Source: CAD feature listing. Evaluate the final solid. Frame: model axes, mm. Coordinates: 2 decimals unless noted, no trailing zeros. Loops run counter-clockwise (first coordinate to the right, second up) from the corner with the lowest first, then second, coordinate; pieces in that order, holes last. Notation, with made-up numbers: (-30, 82.5) -> (-9, 82.5) arc R22 cw to (-9, 102.5) -> close; hole circle Ø8 at (-18, 63). An arc over 180 degrees is marked (long way). One line per question, with ' | ' between items. Start each with the question number.
```python
from build123d import *

# Parameters (mm, degrees)
SKETCH1_W           = 25
SKETCH1_H           = 25
BOSS_EXTRUDE1_DEPTH = 2
SKETCH4_R           = 1.125
BOSS_EXTRUDE3_DEPTH = 0.7
SKETCH5_W           = 21.3
SKETCH5_H           = 21.3
BOSS_EXTRUDE4_DEPTH = 0.01
FILLET1_R           = 0.7
CHAMFER1_SIZE       = 0.5
CUT_EXTRUDE1_DEPTH  = 18.790446875
SKETCH7_R           = 0.4
BOSS_EXTRUDE5_DEPTH = 2


with BuildPart() as part:
    # Sketch1 → Boss-Extrude1 (new body)
    with BuildSketch(Plane.XY):
        Rectangle(SKETCH1_W, SKETCH1_H)
    extrude(amount=BOSS_EXTRUDE1_DEPTH)

    # Sketch4 → Boss-Extrude3 (add)
    with BuildSketch(Plane.XY.offset(2)):
        with Locations((0, 2.5)):
            Circle(SKETCH4_R)
    extrude(amount=BOSS_EXTRUDE3_DEPTH)

    # Sketch5 → Boss-Extrude4 (add)
    with BuildSketch(Plane.XY.offset(2)):
        Rectangle(SKETCH5_W, SKETCH5_H)
    extrude(amount=BOSS_EXTRUDE4_DEPTH)

    # Fillet1
    # the kernel refuses this fillet: 0.7 mm, written as the material it adds along each edge
    with BuildSketch(Plane(origin=(0, 2.5, 2.01), x_dir=(1, 0, 0), z_dir=(0, 1, 0))) as fillet1_piece_1_section:
        with BuildLine():
            CenterArc((1.125 + FILLET1_R, -FILLET1_R), FILLET1_R, 90, 90)
            Line((1.125, -FILLET1_R), (1.125, 0))
            Line((1.125, 0), (1.125 + FILLET1_R, 0))
        make_face()
    fillet1_piece_1 = revolve(axis=Axis((0, 2.5, 2.01), (0, 0, -1)), mode=Mode.PRIVATE)
    fillet1_piece_1 = split(fillet1_piece_1, bisect_by=Plane(origin=(-1.326537578, 2.5, 2.7), z_dir=(0, 0, -1)), keep=Keep.TOP, mode=Mode.PRIVATE)
    add(fillet1_piece_1)

    # Chamfer1
    chamfer1_edges = [part.edges().sort_by_distance(p)[0] for p in [
        (-10.65, -10.65, 2.005),
        (10.65, 10.65, 2.005),
    ]]
    chamfer(chamfer1_edges, length=CHAMFER1_SIZE)

    # Sketch6 → Cut-Extrude1 (cut, through all)
    with BuildSketch(Plane.XY.offset(2)):
        with BuildLine():
            Line((12.5, 9.98277308), (12.5, 12.5))
            Line((12.5, 12.5), (9.98277308, 12.5))
            ThreePointArc((9.98277308, 12.5), (11.762721305, 11.762721305), (12.5, 9.98277308))
        make_face()
        with BuildLine():
            Line((-9.98277308, 12.5), (-12.5, 12.5))
            Line((-12.5, 12.5), (-12.5, 9.98277308))
            ThreePointArc((-12.5, 9.98277308), (-11.762721305, 11.762721305), (-9.98277308, 12.5))
        make_face()
        with BuildLine():
            Line((-12.5, -9.98277308), (-12.5, -12.5))
            Line((-12.5, -12.5), (-9.98277308, -12.5))
            ThreePointArc((-9.98277308, -12.5), (-11.762721305, -11.762721305), (-12.5, -9.98277308))
        make_face()
        with BuildLine():
            Line((12.5, -9.98277308), (12.5, -12.5))
            Line((12.5, -12.5), (9.98277308, -12.5))
            ThreePointArc((9.98277308, -12.5), (11.762721305, -11.762721305), (12.5, -9.98277308))
        make_face()
    extrude(amount=-CUT_EXTRUDE1_DEPTH, mode=Mode.SUBTRACT)

    # Sketch7 → Boss-Extrude5 (add)
    with BuildSketch(Plane(origin=(0, 0, 0), x_dir=(-1, 0, 0), z_dir=(0, 0, -1))):
        with Locations(Location((0, 2.5, 0), (0, 0, 180))):
            Circle(SKETCH7_R)
    extrude(amount=BOSS_EXTRUDE5_DEPTH)


solid = part.part
```
(1) Cut plane A-A, the plane y = 2.5. Return the cut outline in (x, z) (3 decimals).
(2) Cut plane C-C, the plane z = -1.15. Return the cut outline in (x, y), and give its area (3 significant figures).
(3) Cut plane B-B, the plane x = 0. Return the cut outline in (y, z) (3 decimals), and give its area (3 significant figures).
(4) Contact query for a flat-ended pin moving along its axis: pin 1 Ø6 at (x, y) = (2.5, -8) entering from -Z. Output: stop coordinate, or through.
(5) Ray query, L1, parallel to Z at x = -3.75, y = 2.5; L2, parallel to Z at x = 0.5, y = 1.75; L3, parallel to X at y = 10.5, z = 0.3. Return the intervals inside material, ascending.
Here are the results:
1) outline: (-12.5, 0) -> (-0.4, 0) -> (-0.4, -2) -> (0.4, -2) -> (0.4, 0) -> (12.5, 0) -> (12.5, 2) -> (10.65, 2) -> (10.65, 2.01) -> (1.825, 2.01) arc R0.7 cw to (1.125, 2.7) -> (-1.125, 2.7) arc R0.7 cw to (-1.825, 2.01) -> (-10.65, 2.01) -> (-10.65, 2) -> (-12.5, 2) -> close
2) outline: circle Ø0.8 at (0, 2.5) | area: 0.503 mm2
3) outline: (-12.5, 0) -> (2.1, 0) -> (2.1, -2) -> (2.9, -2) -> (2.9, 0) -> (12.5, 0) -> (12.5, 2) -> (10.65, 2) -> (10.65, 2.01) -> (4.325, 2.01) arc R0.7 cw to (3.625, 2.7) -> (1.375, 2.7) arc R0.7 cw to (0.675, 2.01) -> (-10.65, 2.01) -> (-10.65, 2) -> (-12.5, 2) -> close | area: 53.6 mm2
4) pin 1: stops at z = 0
5) L1: z = 0 to 2.01 | L2: z = 0 to 2.7 | L3: x = -12.45 to 12.45
